Design review of the part shown in the three views and the two pictorial views. Dimensions are in mm from the part's minimum x, y and z. A direction names the side the tool comes from. Round coordinates to 2 decimals unless told otherwise and drop trailing zeros. Loops run counter-clockwise (first coordinate to the right, second up) from the corner with the lowest first, then second, coordinate; pieces in that order, holes last. Notation, with made-up numbers: M 0.25,38 L 30.25,38 A28 ccw 30.25,64 Z; hole C 75,59.25 d6. An arc over 180 degrees is marked long. One line per question, with ' | ' between items.
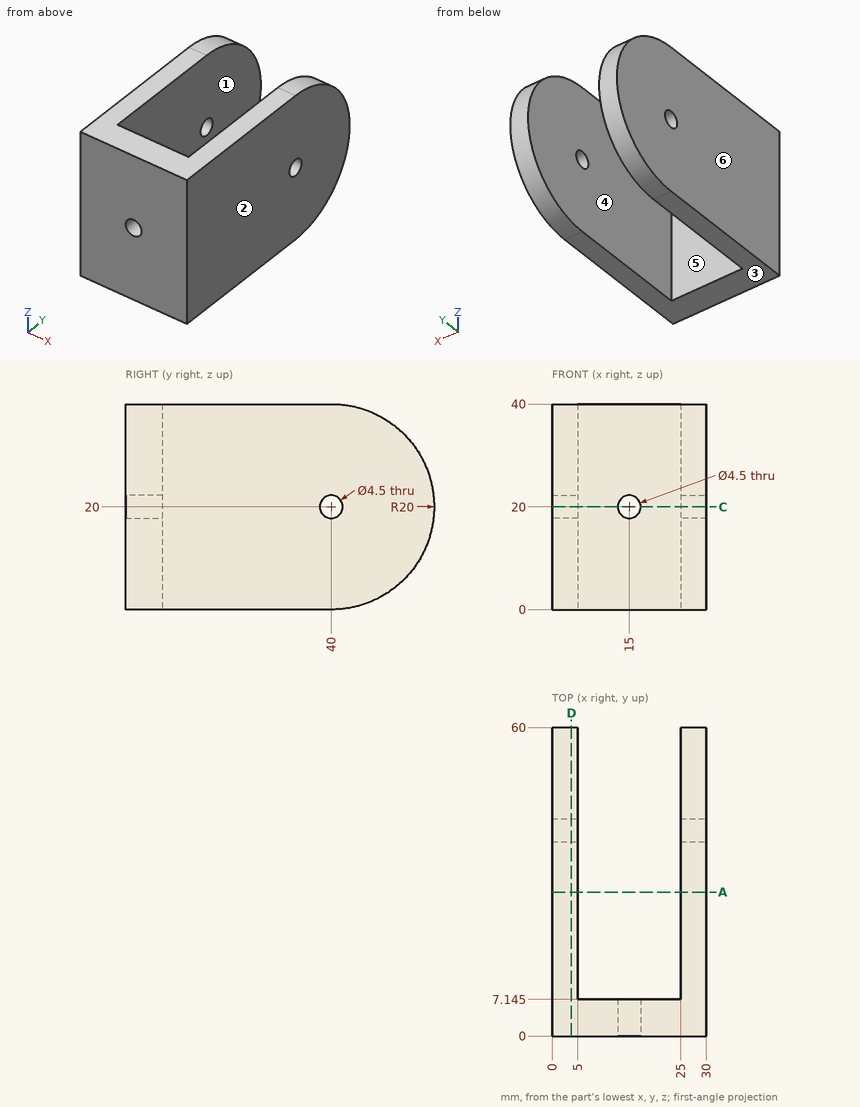
1) Add section D-D on x = 3.75. State the section outline as (y, z) points.
Output values:
outline: M 0,0 L 40,0 A20 ccw 40,40 L 0,40 Z; hole C 40,20 d4.5
2) Machinability: for the marked faces 5 and 6, which of the approach directions +Z, -Z, +X, -X, +Y, -Y give a long, thin tool a straight path to every point of the face, cutting with its end or side? Answer none if there is none.
Output values:
face 5: +Z, -Z, +Y | face 6: +Z, -Z, -X, +Y, -Y
3) Add section C-C on z = 20. State how many separate pieces and enclosed holes the cut face has, then the cut area to 3 significant figures.
Output values:
separate pieces: 4 | enclosed holes: 0 | area: 666 mm²
4) For line 1 (X direction, y = 52, z = 15); line 2 (X direction, y = 2.25, z = 20); line 3 (Y direction, x = 3.55, z = 20), list the stretches that pass through material, from the lowest coordinate up.
Output values:
line 1: x = 0 to 5, 25 to 30 | line 2: x = 0 to 12.75, 17.25 to 30 | line 3: y = 0 to 37.75, 42.25 to 60
5) Insertion check: P1, Ø10, axis at x = 16, y = 41.5, coming from the +Z side; P2, Ø2, axis at x = 24.5, z = 15.5, coming from the +Y side; P3, Ø10, axis at x = 11.5, z = 24.5, coming from the +Y side (3 decimals). Each pin has a flat end and moves straight along its axis. Give the tip position at first contact, or say it passes through.
Output values:
P1: passes through | P2: stops at y = 59.67 | P3: stops at y = 7.145
6) Mouldability with a two-part tool opening along X and no side actions: class the marked faces 1, 2, 3 and 4 as +X half, -X half, draft (parallel to the pull), parting line (faces both ways), or undercut.
Output values:
face 1: undercut | face 2: +X half | face 3: draft | face 4: undercut
7) Add section A-A on y = 28. State the section outline as (x, z) points.
Output values:
outline: M 0,0 L 5,0 L 5,40 L 0,40 Z; M 25,0 L 30,0 L 30,40 L 25,40 Z
